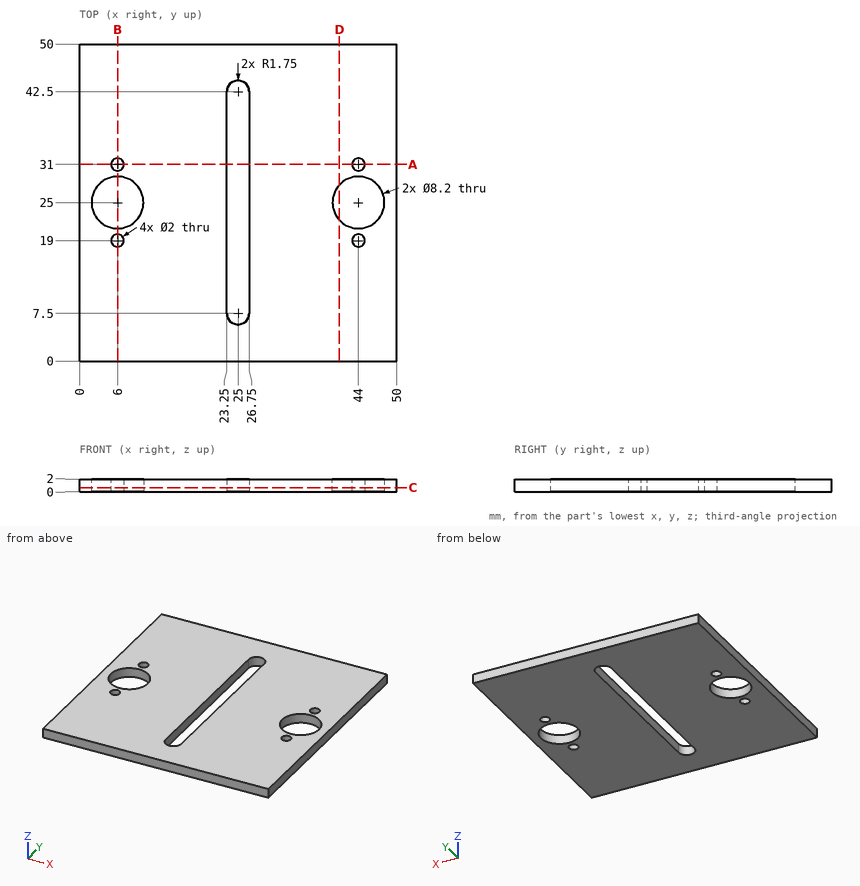
Part print with two shaded views. Sizes in mm from the minimum x, y, z corner. Round coordinates to 2 decimals unless told otherwise and drop trailing zeros. Order: outer loops, then holes, each group sorted by start corner. A loop starts at its lowest first (then second) coordinate and runs counter-clockwise, first axis right, second up. Notation, with made-up numbers: (35.25, -37.5) - (78.25, -37.5) arc R31 ccw to (78.25, -5.5) - close; hole circle Ø8 at (-12.75, -21.5). An arc over 180 degrees is marked (long way). Answer in a Markdown table with one row per item. Add a question column.
(1) Band-saw the part on B-B on x = 6. List the corners of the cut face in (y, z).
(2) Band-saw the part on C-C on z = 0.65. List the corners of the cut face in (x, y).
(3) Band-saw the part on A-A on y = 31. List the corners of the cut face in (x, z), and give its area (3 significant figures).
(4) Probe L1, parallel to Y at x = 44, z = 0.8; L2, parallel to X at y = 28, z = 1.8; L3, parallel to X at y = 26.5, z = 1.15. List the from-to ranges inside material, lowest first. Write a range as [from, to].
(5) Band-saw the part on D-D on x = 41. List the corners of the cut face in (y, z), and give its area (3 significant figures).
Data:
| question | item | result |
|---|---|---|
| 1 | outline | (0, 0) - (18, 0) - (18, 2) - (0, 2) - close; (20, 0) - (20.9, 0) - (20.9, 2) - (20, 2) - close; (29.1, 0) - (30, 0) - (30, 2) - (29.1, 2) - close; (32, 0) - (50, 0) - (50, 2) - (32, 2) - close |
| 2 | outline | (0, 0) - (50, 0) - (50, 50) - (0, 50) - close; hole circle Ø8.2 at (6, 25); hole circle Ø2 at (6, 19); hole circle Ø2 at (6, 31); hole (23.25, 7.5) arc R1.75 ccw to (26.75, 7.5) - (26.75, 42.5) arc R1.75 ccw to (23.25, 42.5) - close; hole circle Ø8.2 at (44, 25); hole circle Ø2 at (44, 19); hole circle Ø2 at (44, 31) |
| 3 | outline | (0, 0) - (5, 0) - (5, 2) - (0, 2) - close; (7, 0) - (23.25, 0) - (23.25, 2) - (7, 2) - close; (26.75, 0) - (43, 0) - (43, 2) - (26.75, 2) - close; (45, 0) - (50, 0) - (50, 2) - (45, 2) - close |
| 3 | area | 85.0 mm^2 |
| 4 | L1 | y = [0, 18], [20, 20.9], [29.1, 30], [32, 50] |
| 4 | L2 | x = [0, 3.21], [8.79, 23.25], [26.75, 41.21], [46.79, 50] |
| 4 | L3 | x = [0, 2.18], [9.82, 23.25], [26.75, 40.18], [47.82, 50] |
| 5 | outline | (0, 0) - (22.21, 0) - (22.21, 2) - (0, 2) - close; (27.79, 0) - (50, 0) - (50, 2) - (27.79, 2) - close |
| 5 | area | 88.8 mm^2 |
